Can you work these out from the model? Positions are in its coordinate system, mm. A direction names the side the tool comes from. Give positions to 0.01 mm unless a question says otherwise; leave off trailing zeros. Write each loop counter-clockwise with the first axis right and the second up, starting at its lowest first coordinate (ties: lowest second). Pieces come first, ordered by that corner, then holes.
from build123d import *

# Parameters (mm, degrees)
F1_DEPTH = 12.5
F2_R     = 5


# Not quite as in the source:
# - a feature names something its author has since deleted; it is built from what else it names


with BuildPart() as f1:
    # F0 (on Front) → F1 (new body, symmetric)
    with BuildSketch(Plane.XZ):
        with BuildLine():
            ThreePointArc((-6.2894771713, 32.5883566917), (0, 37.1817581393), (6.2894771713, 32.5883566917))
            Line((6.2894771713, 32.5883566917), (16.7, 0))
            Line((16.7, 0), (20.7, 0))
            ThreePointArc((20.7, 0), (20.6522901201, 0.6159568218), (20.5102985969, 1.2172200305))
            Line((20.5102985969, 1.2172200305), (11.4429113124, 29.6011211997))
            ThreePointArc((11.4429113124, 29.6011211997), (11.8429318518, 39.3121369153), (18.4103098825, 46.4768691826))
            Line((18.4103098825, 46.4768691826), (53.1603869456, 64.5016425675))
            Line((53.1603869456, 64.5016425675), (65.7802901999, 71.0475531243))
            Line((65.7802901999, 71.0475531243), (63.4780788017, 75.4860013529))
            Line((63.4780788017, 75.4860013529), (-4.8740239191, 40.0319458213))
            ThreePointArc((-4.8740239191, 40.0319458213), (-8.0911004209, 37.4607846039), (-10.0835041229, 33.8565123177))
            Line((-10.0835041229, 33.8565123177), (-20.5102985969, 1.2172200305))
            ThreePointArc((-20.5102985969, 1.2172200305), (-20.6522901201, 0.6159568218), (-20.7, 0))
            Line((-20.7, 0), (-16.7, 0))
            Line((-16.7, 0), (-6.2894771713, 32.5883566917))
        make_face()
        Polygon((-16.7, -5.2822484933), (-16.7, 0), (-20.7, 0), (-20.7, -10.5644969866), (-16.7, -10.5644969866), (-16.7, -6.0322484933), align=None)
        Polygon((20.7, 0), (16.7, 0), (16.7, -5.2822484933), (16.7, -6.0322484933), (16.7, -10.5644969866), (20.7, -10.5644969866), align=None)
        with BuildLine():
            Line((65.7802901999, 71.0475531243), (53.1603869456, 64.5016425675))
            ThreePointArc((53.1603869456, 64.5016425675), (60.6653765198, 65.4706764668), (65.7802901999, 71.0475531243))
        make_face()
        Polygon((-14.7, -5.5168885775), (-16.7, -6.0322484933), (-16.7, -10.5644969866), align=None)
        Polygon((16.7, -10.5644969866), (16.7, -6.0322484933), (14.7, -5.4739810377), align=None)
    extrude(amount=F1_DEPTH, both=True)

    # F2
    f2_edges = [f1.edges().sort_by_distance(p)[0] for p in [
        (16.7, 0, -10.564497),
        (-16.7, 0, -10.564497),
    ]]
    fillet(f2_edges, radius=F2_R)


solid = f1.part
(1) If we mould it in two halves opening along Z, with no side actions, what happens to faces 1 (the face through (-8.05, -0.18, 37.51)), 2 (the face through (10, 12.5, 36)), 3 (the face through (-11.568, -0.175, 16.066)), 4 (the face through (60.57, -0.18, 65.42))? For each: +Z half, -Z half, draft (parallel to the pull), parting line (faces both ways), or undercut.
Returned:
face 1: +Z half
face 2: draft
face 3: undercut
face 4: -Z half
(2) Imagine slicing it at C-C, the plane x = 3.5. Write out the boundary of the cut face in (y, z), plus the area to 3 significant figures.
Returned:
outline: (-12.5, 36.18) - (12.5, 36.18) - (12.5, 44.38) - (-12.5, 44.38) - close
area: 205 mm2
(3) For faces 5 (the face through (17.3, -0.2, -9.7)), 6 (the face through (20.7, 0, -5)), 7 (the face through (11.422, -0.175, 16.522)), which set-ups out of +Z, -Z, +X, -X, +Y, -Y let a thin tool reach every point of the face, with its end or its side?
Returned:
face 5: -Z, +Y, -Y
face 6: -Z, +X, +Y, -Y
face 7: +Y, -Y
(4) Imagine slicing it at A-A, the plane z = -2. Write out the boundary of the cut face in (x, y), plus the area to 3 significant figures.
Returned:
outline: (-20.7, -12.5) - (-16.7, -12.5) - (-16.7, 12.5) - (-20.7, 12.5) - close; (16.7, -12.5) - (20.7, -12.5) - (20.7, 12.5) - (16.7, 12.5) - close
area: 200 mm2
(5) Imagine slicing it at B-B, the plane y = 5.25. Write out the boundary of the cut face in (x, z), plus the area to 3 significant figures.
Returned:
outline: (-20.7, -10.56) - (-20.1, -10.56) arc R5 ccw to (-15.45, -7.41) - (-14.7, -5.52) - (-16.7, -6.03) - (-16.7, 0) - (-6.29, 32.59) arc R6.6 cw to (6.29, 32.59) - (16.7, 0) - (16.7, -6.03) - (14.7, -5.47) - (15.45, -7.39) arc R5 ccw to (20.11, -10.56) - (20.7, -10.56) - (20.7, 0) arc R4 ccw to (20.51, 1.22) - (11.44, 29.6) arc R14.16 cw to (18.41, 46.48) - (53.16, 64.5) arc R11.03 ccw to (65.78, 71.05) - (63.48, 75.49) - (-4.87, 40.03) arc R10.59 ccw to (-10.08, 33.86) - (-20.51, 1.22) arc R4 ccw to (-20.7, 0) - close
area: 869 mm2
(6) If I drill on L1, parallel to X at y = -5.25, z = -5; L2, parallel to X at y = -5, z = 9; L3, parallel to Z at x = 57, y = -0.75, over which ranges is the centre line in solid material (lowest first)?
Returned:
L1: x = -20.7 to -16.7, 16.7 to 20.7
L2: x = -18.02 to -13.82, 13.82 to 18.02
L3: z = 64.32 to 72.13
(7) Imagine slicing it at D-D, the plane z = 7. Write out the boundary of the cut face in (x, y).
Returned:
outline: (-18.66, -12.5) - (-14.46, -12.5) - (-14.46, 12.5) - (-18.66, 12.5) - close; (14.46, -12.5) - (18.66, -12.5) - (18.66, 12.5) - (14.46, 12.5) - close
(8) Will these pins go through, and if not, where does the flat tip stop? P1, Ø3, axis at y = 6.5, z = 32, coming from the -X side; P2, Ø4, axis at y = 9.5, z = 53.5, coming from the -X side; P3, Ø1.8, axis at y = -0.5, z = -4.5, coming from the +X side.
Returned:
P1: stops at x = -11.16
P2: stops at x = 17.24
P3: stops at x = 20.7
